```python
from build123d import *

# Parameters (mm, degrees)
F0_W          = 73.025
F0_H          = 15.875
F1_DEPTH      = 9.525
F1_DEPTH_BACK = 6.35
F2_R          = 5.1435
F3_DEPTH      = 9.525
F4_R          = 3.175
F5_DEPTH      = 57.15
F6_R          = 3.96875
F7_DEPTH      = 9.525


with BuildPart() as f1:
    # F0 (on Front) → F1 (new body, two sides)
    with BuildSketch(Plane.XZ) as f1_sk:
        Rectangle(F0_W, F0_H)
    extrude(amount=F1_DEPTH)
    extrude(f1_sk.sketch, amount=-F1_DEPTH_BACK)

    # F2 (on face) → F3 (cut)
    with BuildSketch(Plane(origin=(-36.5125, 0, 0), x_dir=(0, -1, 0), z_dir=(-1, 0, 0))):
        Circle(F2_R)
    extrude(amount=-F3_DEPTH, mode=Mode.SUBTRACT)

    # F4 (on face) → F5 (cut)
    with BuildSketch(Plane(origin=(-36.5125, 0, 0), x_dir=(0, -1, 0), z_dir=(-1, 0, 0))):
        Circle(F4_R)
    extrude(amount=-F5_DEPTH, mode=Mode.SUBTRACT)

    # F6 (on face) → F7 (cut, through all)
    with BuildSketch(Plane.XZ.offset(9.525)):
        with Locations((-3.937, 0)):
            Circle(F6_R)
        with Locations((-19.8374, 0)):
            Circle(F6_R)
        with Locations((11.9634, 0)):
            Circle(F6_R)
        with Locations((27.8638, 0)):
            Circle(F6_R)
    extrude(amount=-F7_DEPTH, mode=Mode.SUBTRACT)


solid = f1.part
```
Geometry check sheet. Reference: the model listing, model coordinates, mm. A direction names the side the tool comes from. Give positions to 0.01 mm unless a question says otherwise; leave off trailing zeros. Loops run counter-clockwise (first coordinate to the right, second up) from the corner with the lowest first, then second, coordinate; pieces in that order, holes last. Notation, with made-up numbers: (-40, 52.5) - (-26, 52.5) arc R28 cw to (-26, 78.5) - close; hole circle Ø10 at (-31, 46). An arc over 180 degrees is marked (long way). Use CSV: the item, a comma, the result in double quotes. Start each with the question number.
Q1. Access from +Z, -Z, +X, -X, +Y, -Y to the whole of each face (thin tool, end or side, straight path). Record for faces 4 (the face through (-1, 6.35, 0)), 5 (the face through (-16.17, -5.89, -1.52)), 6 (the face through (20.637, 0, 0)).
Q2. Section check B-B, the plane y = -8.5. Record the cut outline in (x, z).
Q3. Go/stop test with flat-tipped pins: pin 1 Ø6.5 at (x, z) = (11.96, 0) entering from -Y; pin 2 Ø5 at (y, z) = (0, 1) entering from -X. Record where each tip stops, or that it passes through.
Q4. Scan lines: probe 1 along Z at (x, y) = (-30.25, 0); probe 2 along Z at (x, y) = (-20, -1); probe 3 along X at (y, z) = (-6.25, 1.25). Record each from-to range of solid material in increasing order. Write a range as from..to.
Q5. Release check for a two-part mould opening along Z. For faces 1 (the face through (-31.82, 0.67, 5.1)), 2 (the face through (36.512, -2, 0)), 3 (the face through (-1, -2, -7.938)) record: +Z half, -Z half, draft (parallel to the pull), parting line (faces both ways), or undercut.
Q6. Section check A-A, the plane z = 0. Count the separate pieces of the cut face and the enclosed holes in it, and give its area (3 significant figures).
Findings below:
1,face 4,"+Z, -Z, +X, -X, +Y"
1,face 5,"-Y"
1,face 6,"-X"
2,outline,"(-36.51, -7.94) - (36.51, -7.94) - (36.51, 7.94) - (-36.51, 7.94) - close; hole circle Ø7.94 at (-19.84, 0); hole circle Ø7.94 at (-3.94, 0); hole circle Ø7.94 at (11.96, 0); hole circle Ø7.94 at (27.86, 0)"
3,pin 1,"stops at y = 0"
3,pin 2,"stops at x = -26.99"
4,probe 1,"z = -7.94..-5.14, 5.14..7.94"
4,probe 2,"z = -7.94..-3.97, 3.97..7.94"
4,probe 3,"x = -36.51..-23.6, -16.07..-7.7, -0.17..8.2, 15.73..24.1, 31.63..36.51"
5,face 1,"undercut"
5,face 2,"draft"
5,face 3,"-Z half"
6,separate pieces,"4"
6,enclosed holes,"0"
6,area,"532 mm^2"
